Verification items for this drawing (mm, ordinates from the low corner). A direction names the side the tool comes from. Coordinates: 2 decimals unless noted, no trailing zeros. Loops run counter-clockwise (first coordinate to the right, second up) from the corner with the lowest first, then second, coordinate; pieces in that order, holes last.
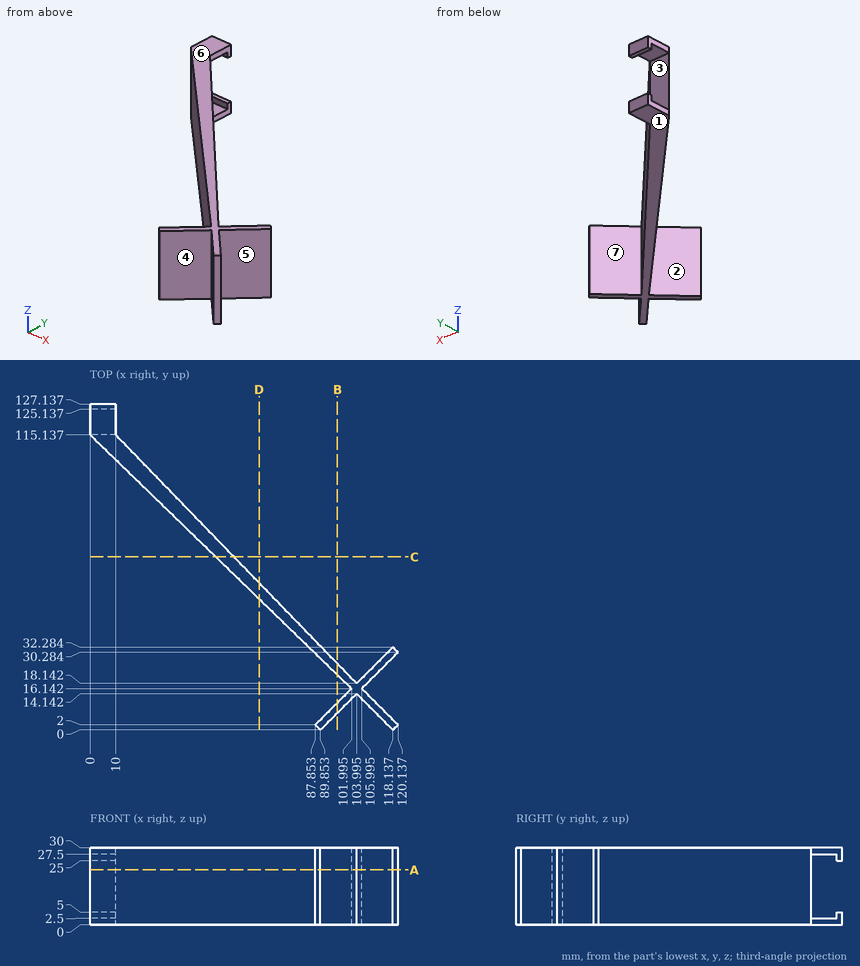
(1) Section check D-D, the plane x = 66. Enter the section's corners in (y, z).
(2) Scan lines: line 1 along Y through (x, z) = (90.5, 20.75); line 2 along Y through (x, z) = (5.5, 4); line 3 along X through (y, z) = (31, 16) (1 decimal). Record each from-to range of solid material in increasing order.
(3) Gauge pin test, flat ends, axial feed: P1, Ø2, axis at x = 3.5, z = 25.5, coming from the -Y side; P2, Ø8, axis at x = 4.5, z = 12, coming from the +Y side; P3, Ø1, axis at y = 55, z = 22.5, coming from the +X side. Record the tip position at first contact, or that the pin passes through.
(4) Section check C-C, the plane y = 67.5. Enter the section's corners in (x, z).
(5) Set-up check for the marked faces 1, 2 and 3: record each of +Z, -Z, +X, -X, +Y, -Y from which the full face is reachable in a straight line by a thin tool's end or side.
(6) Section check B-B, the plane x = 96.5. Enter the section's corners in (y, z) (1 decimal).
(7) Section check A-A, the plane z = 21.5. Enter the section's corners in (x, y) (1 decimal).
(8) Draft check along Y on the marked faces 4, 5, 6 and 7. Enter one of: pulls with the +Y half, pulls with the -Y half, needs draft (parallel to the pull), parting line crosses it, or undercut.
Determined:
1. outline: (51.08, 0) - (57.35, 0) - (57.35, 30) - (51.08, 30) - close
2. line 1: y = 0.65 to 4.65, 27.3 to 32.07
2. line 2: y = 109.8 to 115.14, 125.14 to 127.14
2. line 3: x = 86.7 to 91.5, 116.9 to 119.4
3. P1: stops at y = 110.77
3. P2: stops at y = 115.14
3. P3: stops at x = 68.76
4. outline: (49.08, 0) - (56.16, 0) - (56.16, 30) - (49.08, 30) - close
5. face 1: -Z, +X, -X, +Y, -Y
5. face 2: +Z, -Z, -X
5. face 3: +X, -X
6. outline: (6.6, 0) - (10.6, 0) - (10.6, 30) - (6.6, 30) - close; (21.5, 0) - (25.9, 0) - (25.9, 30) - (21.5, 30) - close
7. outline: (0, 115.1) - (102, 16.1) - (87.9, 2) - (89.9, 0) - (104, 14.1) - (118.1, 0) - (120.1, 2) - (106, 16.1) - (120.1, 30.3) - (118.1, 32.3) - (104, 18.1) - (10, 115.1) - close
8. face 4: pulls with the -Y half
8. face 5: undercut
8. face 6: needs draft
8. face 7: pulls with the +Y half
